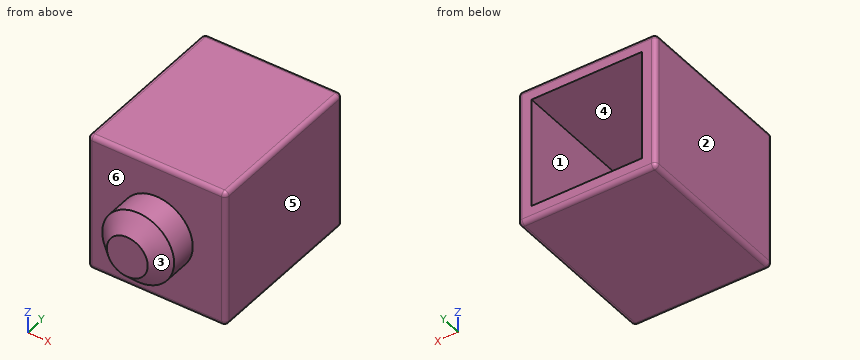
from build123d import *

# Parameters (mm, degrees)
F0_W     = 15.875
F0_H     = 15.875
F1_DEPTH = 19.05
F2_R     = 4.1275
F3_DEPTH = 4.826
F4_SIZE  = 1.778
F5_T     = -1.5875
F6_R     = 0.508


with BuildPart() as f1:
    # F0 (on Front) → F1 (new body)
    with BuildSketch(Plane.XZ):
        Rectangle(F0_W, F0_H)
    extrude(amount=F1_DEPTH)

    # F2 (on face) → F3 (join)
    with BuildSketch(Plane.XZ.offset(19.05)):
        Circle(F2_R)
    extrude(amount=F3_DEPTH)

    # F4
    f4_edges = [f1.edges().sort_by_distance(p)[0] for p in [
        (-4.1275, -23.876, 0),
    ]]
    chamfer(f4_edges, length=F4_SIZE)

    # F5
    f5_openings = [f1.faces().sort_by_distance(p)[0] for p in [
        (0, 0, 0),
    ]]
    offset(amount=F5_T, openings=f5_openings, kind=Kind.INTERSECTION)

    # F6
    f6_edges = [f1.edges().sort_by_distance(p)[0] for p in [
        (0, -19.05, 7.9375),
        (-7.9375, -19.05, 0),
        (0, -19.05, -7.9375),
        (7.9375, -19.05, 0),
        (-7.9375, -9.525, 7.9375),
        (-7.9375, -9.525, -7.9375),
        (7.9375, -9.525, 7.9375),
        (7.9375, -9.525, -7.9375),
        (0, 0, -7.9375),
        (7.9375, 0, 0),
        (0, 0, 7.9375),
        (-7.9375, 0, 0),
    ]]
    fillet(f6_edges, radius=F6_R)


solid = f1.part
Build history of the part. All positions in model axes, mm. Face numbers are marked on the shaded views. A direction names the side the tool comes from. Give positions to 0.01 mm unless a question says otherwise; leave off trailing zeros. Order: outer loops, then holes, each group sorted by start corner. A loop starts at its lowest first (then second) coordinate and runs counter-clockwise, first axis right, second up. Notation, with made-up numbers: M 83,-32.5 L 132,-32.5 A22 cw 132,-0.5 Z; hole C 71,-4 d6. An arc over 180 degrees is marked long. Put each result on its own line as item: value.
Item 1: Cut at A-A on y = -4. Write the cut outline in (x, z).
Results are:
outline: M -7.94,-7.43 A0.51 ccw -7.43,-7.94 L 7.43,-7.94 A0.51 ccw 7.94,-7.43 L 7.94,7.43 A0.51 ccw 7.43,7.94 L -7.43,7.94 A0.51 ccw -7.94,7.43 Z; hole M -6.35,-6.35 L 6.35,-6.35 L 6.35,6.35 L -6.35,6.35 Z
Item 2: Wall check: probe 1 along Z at (x, y) = (5.75, -11.75). Give the ranges that are in metal, low to high.
Results are:
probe 1: -7.94 to -6.35, 6.35 to 7.94
Item 3: Cut at B-B on z = 4.5. Write the cut outline in (x, y), then the cut area to 3 significant figures.
Results are:
outline: M -7.94,-18.54 A0.51 ccw -7.43,-19.05 L 7.43,-19.05 A0.51 ccw 7.94,-18.54 L 7.94,-0.51 A0.51 ccw 7.43,0 L 6.35,0 L 6.35,-17.46 L -6.35,-17.46 L -6.35,0 L -7.43,0 A0.51 ccw -7.94,-0.51 Z
area: 80.4 mm2
Item 4: Drop a flat-ended pin along its axis: pin 1 Ø1.7 at (x, z) = (0.5, -0.5) entering from +Y. Give the stop position or say it passes through.
Results are:
pin 1: y = -22.29
Item 5: Cut at D-D on z = 0. Write the cut outline in (x, y), then the cut area to 3 significant figures.
Results are:
outline: M -7.94,-18.54 A0.51 ccw -7.43,-19.05 L -4.13,-19.05 L -4.13,-22.1 L -2.35,-23.88 L 2.35,-23.88 L 4.13,-22.1 L 4.13,-19.05 L 7.43,-19.05 A0.51 ccw 7.94,-18.54 L 7.94,-0.51 A0.51 ccw 7.43,0 L 6.35,0 L 6.35,-17.46 L 2.54,-17.46 L 2.54,-21.44 L 1.69,-22.29 L -1.69,-22.29 L -2.54,-21.44 L -2.54,-17.46 L -6.35,-17.46 L -6.35,0 L -7.43,0 A0.51 ccw -7.94,-0.51 Z
area: 93.3 mm2
Item 6: Which spindle directions (+Z, -Z, +X, -X, +Y, -Y) get a long thin tool onto all of the face, cutting with end or side? Do the marked faces 5 and 6. Say none if no direction does.
Results are:
face 5: +Z, -Z, +X, +Y, -Y
face 6: -Y
Item 7: Pull direction Z, two halves, no side cores. Call the marked faces 1, 2, 3 and 4: +Z half, -Z half, draft (parallel to the pull), parting line (faces both ways), or undercut.
Results are:
face 1: undercut
face 2: draft
face 3: parting line
face 4: undercut
Item 8: Cut at C-C on x = 0. Write the cut outline in (y, z), then the cut area to 3 significant figures.
Results are:
outline: M -23.88,-2.35 L -22.1,-4.13 L -19.05,-4.13 L -19.05,-7.43 A0.51 ccw -18.54,-7.94 L -0.51,-7.94 A0.51 ccw 0,-7.43 L 0,-6.35 L -17.46,-6.35 L -17.46,-2.54 L -21.44,-2.54 L -22.29,-1.69 L -22.29,1.69 L -21.44,2.54 L -17.46,2.54 L -17.46,6.35 L 0,6.35 L 0,7.43 A0.51 ccw -0.51,7.94 L -18.54,7.94 A0.51 ccw -19.05,7.43 L -19.05,4.13 L -22.1,4.13 L -23.88,2.35 Z
area: 93.3 mm2
